Geometry check sheet. Reference: the model listing, model coordinates, mm. A direction names the side the tool comes from. Give positions to 0.01 mm unless a question says otherwise; leave off trailing zeros. Write each loop counter-clockwise with the first axis right and the second up, starting at its lowest first coordinate (ties: lowest second). Pieces come first, ordered by that corner, then holes. Notation, with made-up numbers: (67.5, -24) -> (100.5, -24) arc R15 ccw to (100.5, -17) -> close; hole circle Ø2 at (56, 58). An arc over 180 degrees is marked (long way). One line per item, written item: value.
from build123d import *

# Parameters (mm, degrees)
SKETCH2_W           = 52
SKETCH2_H           = 9.5
SKETCH2_W_2         = 46
SKETCH2_H_2         = 3.5
BOSS_EXTRUDE1_DEPTH = 3
FILLET1_R           = 2
FILLET2_R           = 1


with BuildPart() as part:
    # Sketch2 → Boss-Extrude1 (new body)
    with BuildSketch(Plane(origin=(0, 0, 0), x_dir=(1, 0, 0), z_dir=(0, 1, 0))):
        with Locations((10.397099769, -9.98104869)):
            Rectangle(SKETCH2_W, SKETCH2_H)
        with Locations((10.397099769, -9.98104869)):
            Rectangle(SKETCH2_W_2, SKETCH2_H_2, mode=Mode.SUBTRACT)
    extrude(amount=BOSS_EXTRUDE1_DEPTH)

    # Fillet1
    # the kernel refuses this fillet: 2 mm, written as the material it adds along each edge
    with BuildSketch(Plane(origin=(33.397099769, 0, 11.73104869), x_dir=(-1, 0, 0), z_dir=(0, 1, 0)), Plane(origin=(33.397099769, 0, 8.23104869), x_dir=(0, 0, 1), z_dir=(0, 1, 0)), Plane(origin=(-12.602900231, 0, 11.73104869), x_dir=(0, 0, -1), z_dir=(0, 1, 0))) as fillet1_piece_1:
        with BuildLine():
            CenterArc((FILLET1_R, -FILLET1_R), FILLET1_R, 90, 90)
            Line((0, -FILLET1_R), (0, 0))
            Line((0, 0), (FILLET1_R, 0))
        make_face()
    extrude(amount=3)
    with BuildSketch(Plane(origin=(-12.602900231, 0, 8.23104869), x_dir=(0, 0, 1), z_dir=(0, 1, 0))) as fillet1_piece_2:
        with BuildLine():
            CenterArc((FILLET1_R, FILLET1_R), FILLET1_R, 180, 90)
            Line((0, FILLET1_R), (0, 0))
            Line((0, 0), (FILLET1_R, 0))
        make_face()
    extrude(amount=3)

    # Fillet2
    fillet2_edges = [part.edges().sort_by_distance(p)[0] for p in [
        (36.397099769, 3, 9.98104869),
        (10.397099769, 3, 5.23104869),
        (-15.602900231, 3, 9.98104869),
        (10.397099769, 0, 5.23104869),
        (36.397099769, 0, 9.98104869),
        (10.397099769, 0, 14.73104869),
        (-15.602900231, 0, 9.98104869),
        (-15.602900231, 1.5, 5.23104869),
        (36.397099769, 1.5, 5.23104869),
        (36.397099769, 1.5, 14.73104869),
        (-15.602900231, 1.5, 14.73104869),
        (10.397099769, 3, 14.73104869),
    ]]
    fillet(fillet2_edges, radius=FILLET2_R)


solid = part.part
1) Tool access check on faces 1 (the cylindrical face through (36.1, 2.71, 9.93)), 2 (the flat face through (10, 1, 8.231)). Record the directions out of +Z, -Z, +X, -X, +Y, -Y that give a thin tool (end or side, any length) a straight path to the whole face; none if there is none.
Verdict:
face 1: +Z, -Z, +X, +Y
face 2: +Y, -Y
2) Mould release check, pull along X, two halves, no side actions. Record for faces 3 (the flat face through (10, 1, 11.731)), 4 (the cylindrical face through (10.747, 2.715, 14.43)), 5 (the flat face through (36.397, 1.5, 10)): released by +X, released by -X, zero draft, split by the parting line, or undercut.
Verdict:
face 3: undercut
face 4: zero draft
face 5: released by +X
3) Sectioned sample at B-B on y = 1.45. Record the cut outline in (x, z).
Verdict:
outline: (-15.6, 6.23) arc R1 ccw to (-14.6, 5.23) -> (35.4, 5.23) arc R1 ccw to (36.4, 6.23) -> (36.4, 13.73) arc R1 ccw to (35.4, 14.73) -> (-14.6, 14.73) arc R1 ccw to (-15.6, 13.73) -> close; hole (-12.59, 9.98) arc R2 ccw to (-10.6, 8.23) -> (31.4, 8.23) arc R2 ccw to (33.38, 9.98) arc R2 ccw to (31.4, 11.73) -> (-10.6, 11.73) arc R2 ccw to start
4) Sectioned sample at C-C on z = 10.5. Record the cut outline in (x, y), plus the area to 3 significant figures.
Verdict:
outline: (-15.6, 1) arc R1 ccw to (-14.6, 0) -> (-12.45, 0) -> (-12.45, 3) -> (-14.6, 3) arc R1 ccw to (-15.6, 2) -> close; (33.24, 0) -> (35.4, 0) arc R1 ccw to (36.4, 1) -> (36.4, 2) arc R1 ccw to (35.4, 3) -> (33.24, 3) -> close
area: 18.1 mm^2
5) Scan lines: probe 1 along X at (y, z) = (1.45, 10); probe 2 along Z at (x, y) = (26, 2.1); probe 3 along X at (y, z) = (2.8, 9.5). Record each from-to range of solid material in increasing order.
Verdict:
probe 1: -15.6 to -12.58, 33.38 to 36.4
probe 2: 5.24 to 8.23, 11.73 to 14.73
probe 3: -15.2 to -12.46, 33.26 to 36
6) Sectioned sample at A-A on x = -10. Record the cut outline in (y, z), plus the area to 3 significant figures.
Verdict:
outline: (0, 6.23) arc R1 ccw to (1, 5.23) -> (2, 5.23) arc R1 ccw to (3, 6.23) -> (3, 8.23) -> (0, 8.23) -> close; (0, 11.73) -> (3, 11.73) -> (3, 13.73) arc R1 ccw to (2, 14.73) -> (1, 14.73) arc R1 ccw to (0, 13.73) -> close
area: 17.1 mm^2
